Autodesk Inventor part; units mm, degrees
ref_plane "Work Plane1" through (41, 0, 0) normal (-1, 0, 0) x (0, 0, 1)
ref_plane "YZ Plane" through (0, 0, 0) normal (1, 0, 0) x (0, 1, 0)
ref_plane "XZ Plane" through (0, 0, 0) normal (0, 1, 0) x (-1, 0, 0)
sketch "Sketch2" plane through (0, 0, 0) normal (1, 0, 0) x (0, 1, 0)
  line L0 (-114, -127.2132) -> (-112.153, -129.5772)
  line L1 (-112.153, -129.5772) -> (84, 23.6743)
  line L2 (-114, -127.2132) -> (-114, -57.4172)
  line L3 (-114, -57.4172) -> (-84, -33.9786)
  circle A0 centre (0, 5) radius 17.5
  circle A1 centre (0, 5) radius 31
  line L4 (-114, -127.2132) -> (84, 27.4814)
  line L5 (84, -40) -> (84, 40)
  line L6 (-84, -40) -> (84, -40)
  line L7 (76.1199, 17.5177) -> (74.2729, 19.8817)
  line L8 (64.2997, 8.2828) -> (62.4527, 10.6468)
  line L9 (-84, 40) -> (-84, -40)
  line L10 (84, 40) -> (-84, 40)
  line L11 (38.2954, -12.034) -> (36.4484, -9.67)
  line L12 (50.1155, -2.7991) -> (48.2686, -0.4351)
  line L13 (12.291, -32.3509) -> (10.444, -29.9868)
  line L14 (24.1112, -23.116) -> (22.2642, -20.7519)
  line L15 (83.212, 23.0587) -> (81.365, 25.4227)
  point P0 (0, 0)
  dimension "d49" = 3
  dimension "d37" = 62
  dimension "d38" = 35
  dimension "d39" = 142
  dimension "d40" = 168
  dimension "d41" = 198
  dimension "d42" = 15
  dimension "d43" = 33
  dimension "d44" = 48
  dimension "d45" = 66
  dimension "d46" = 81
  dimension "d47" = 238.9218
  dimension "d48" = 80
  dimension "d50" = 58
  dimension "d51" = 84
  dimension "d52" = 70.7683
  dimension "d53" = 40
  dimension "d54" = 84
  dimension "d55" = 67.69
  dimension "d56" = 1
extrude "Extrusion1" add sketch "Sketch2" along normal blind 82 contours L4 L6 L1 L0 | L4 L13 L1 L6 | L4 L14 L1 L13 | L4 L11 L1 L14 | L4 L12 L1 L11 | L1 L7 L4 L15 | L4 L8 L1 L12 | L1 L8 L4 L7
extrude "Extrusion2" add sketch "Sketch2" against normal blind 3 contours L4 L14 L1 L13 | L4 L12 L1 L11 | L1 L8 L4 L7
ref_plane "Work Plane1" through (41, 0, 0) normal (-1, 0, 0) x (0, 0, 1)
mirror "Mirror1" about plane through (41, 0, 0) normal (-1, 0, 0) of "Extrusion2"
sketch "Sketch3" plane through (82, 34.1157, -15.2995) normal (0, 0.6156615, -0.7880108) x (-1, 0, 0)
  line L0 (-3, -195.6177) -> (85, -195.6177)
  line L1 (-3, -185.6177) -> (-3, -195.6177)
  line L2 (85, -185.6177) -> (85, -195.6177)
  line L3 (82, -185.6177) -> (82, -27.696)
  line L4 (0, -185.6177) -> (0, -27.696)
  line L5 (82, -185.6177) -> (0, -185.6177)
  line L6 (-3, -185.6177) -> (85, -185.6177)
  dimension "d57" = 10
  dimension "d58" = 3
  dimension "d59" = 3
extrude "Extrusion3" add sketch "Sketch3" against normal up to surface (3 mm away)
fillet "Fillet1" radius 10 2 edges at (85, -120.9566, -134.5518) (-3, -120.9566, -134.5518)
properties part number "Rampa"
Could you check a few things on this model? Use its own coordinates, in mm. A direction names the side the tool comes from. Give positions to 0.01 mm unless a question says otherwise; leave off trailing zeros. Order: outer loops, then holes, each group sorted by start corner. A loop starts at its lowest first (then second) coordinate and runs counter-clockwise, first axis right, second up. Notation, with made-up numbers: (-17, 48.25) - (4, 48.25) arc R31 ccw to (4, 75.25) - close; hole circle Ø2 at (58.25, -36.5). An arc over 180 degrees is marked (long way). One line per item, written item: value. Start each with the question number.
1. Imagine slicing it at C-C on y = -6. List the corners of the cut face in (x, z) for me, plus the area to 3 significant figures.
2. Imagine slicing it at B-B on z = -89.5. List the corners of the cut face in (x, y) for me.
3. For faces 1 (the face through (82, 79, 22)), 2 (the face through (85, 43, -6)), 3 (the face through (0, 79, 22)), which set-ups out of +Z, -Z, +X, -X, +Y, -Y let a thin tool reach every point of the face, with its end or its side?
4. For P1, Ø6, axis at x = 38, z = -73, coming from the +Y side; P2, Ø5, axis at x = 76, y = 62, coming from the -Z side; P3, Ø3, axis at x = 61.5, y = -52.5, coming from the +Z side, each with a flat end and sliding along its axis, tell me the tip position at first contact or that it passes through.
5. If I drill on probe 1 along Y at (x, z) = (9, 10.5); probe 2 along Y at (x, z) = (67, -115); probe 3 along Z at (x, y) = (47, 42), over which ranges is the centre line in solid material (lowest first)?
6. Imagine slicing it at A-A on x = 20. List the corners of the cut face in (y, z) for me (3 decimals).
Values:
1. outline: (0, -46.64) - (82, -46.64) - (82, -42.83) - (0, -42.83) - close
1. area: 312 mm²
2. outline: (0, -65.73) - (82, -65.73) - (82, -60.86) - (0, -60.86) - close
3. face 1: +Z, +X, +Y
3. face 2: +Z, -Z, +X, +Y, -Y
3. face 3: +Z, -X, +Y
4. P1: y = -35.9
4. P2: z = 4.53
4. P3: z = -77.99
5. probe 1: 62.26 to 67.14
5. probe 2: -98.37 to -93.5
5. probe 3: -9.14 to -5.33
6. outline: (-121.88, -133.37) - (-120.033, -135.734) - (12.291, -32.351) - (64.3, 8.283) - (83.212, 23.059) - (81.365, 25.423) - (-114, -127.213) - close
